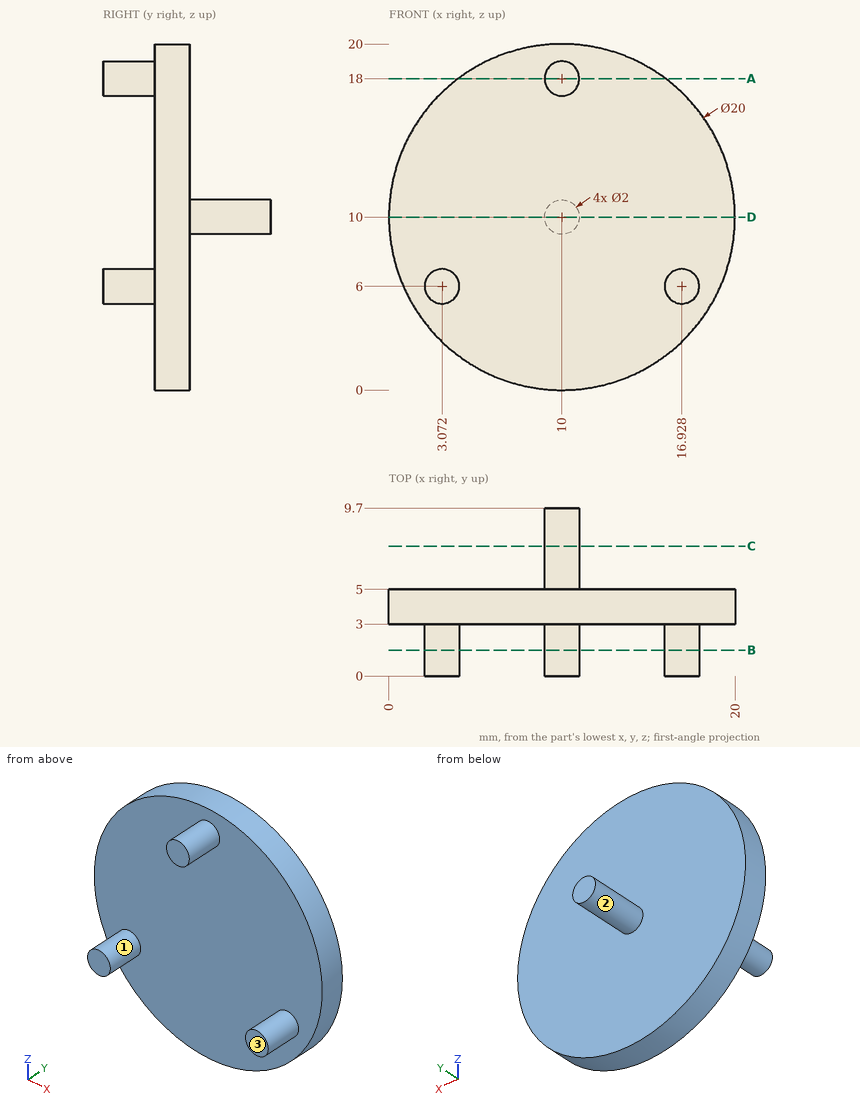
The drawing under review shows one solid part. Ordinate dimensions are in mm from its lowest x, y, z. A direction names the side the tool comes from. Give positions to 0.01 mm unless a question says otherwise; leave off trailing zeros. Loops run counter-clockwise (first coordinate to the right, second up) from the corner with the lowest first, then second, coordinate; pieces in that order, holes last. Notation, with made-up numbers: M 68,51.5 L 81,51.5 A18 cw 81,59.5 Z; hole C 63.25,64 d10. An arc over 180 degrees is marked long. One line per item, written item: value. Start each with the question number.
Q1. Add section A-A (z = 18). Give the boundary of the cut face in (x, y), and give its area (3 significant figures).
Q2. Add section B-B (y = 1.5). Give the boundary of the cut face in (x, z).
Q3. Clearance check with flat-ended pins moving along their axes: pin 1 Ø2 at (x, y) = (7, 7.5) entering from -Z; pin 2 Ø3 at (y, z) = (4.5, 6.5) entering from +X; pin 3 Ø10 at (x, z) = (5, 14) entering from +Y; pin 4 Ø1 at (x, y) = (8.5, 3) entering from +Z. State where each tip first meets the part, or that it passes through.
Q4. Add section D-D (z = 10). Give the boundary of the cut face in (x, y).
Q5. Add section C-C (y = 7.5). Give the boundary of the cut face in (x, z), and give its area (3 significant figures).
Q6. Machinability: for the marked faces 1, 2 and 3, which of the approach directions +Z, -Z, +X, -X, +Y, -Y give a long, thin tool a straight path to every point of the face, cutting with its end or side? Answer none if there is none.
Q7. For L1, parallel to Y at x = 4.5, z = 9.5; L2, parallel to Z at x = 13, y = 4.5; L3, parallel to Z at x = 8.75, y = 4.75, list the stretches that pass through material, from the lowest coordinate up.
Reply:
1. outline: M 4,3 L 9,3 L 9,0 L 11,0 L 11,3 L 16,3 L 16,5 L 4,5 Z
1. area: 30.0 mm²
2. outline: C 3.07,6 d2; C 10,18 d2; C 16.93,6 d2
3. pin 1: through
3. pin 2: x = 19.8
3. pin 3: y = 5
3. pin 4: z = 19.95
4. outline: M 0,3 L 20,3 L 20,5 L 11,5 L 11,9.7 L 9,9.7 L 9,5 L 0,5 Z
5. outline: C 10,10 d2
5. area: 3.14 mm²
6. face 1: -Y
6. face 2: +Y
6. face 3: +Z, -Z, +X, -X, -Y
7. L1: 3 to 5
7. L2: 0.46 to 19.54
7. L3: 0.08 to 19.92
